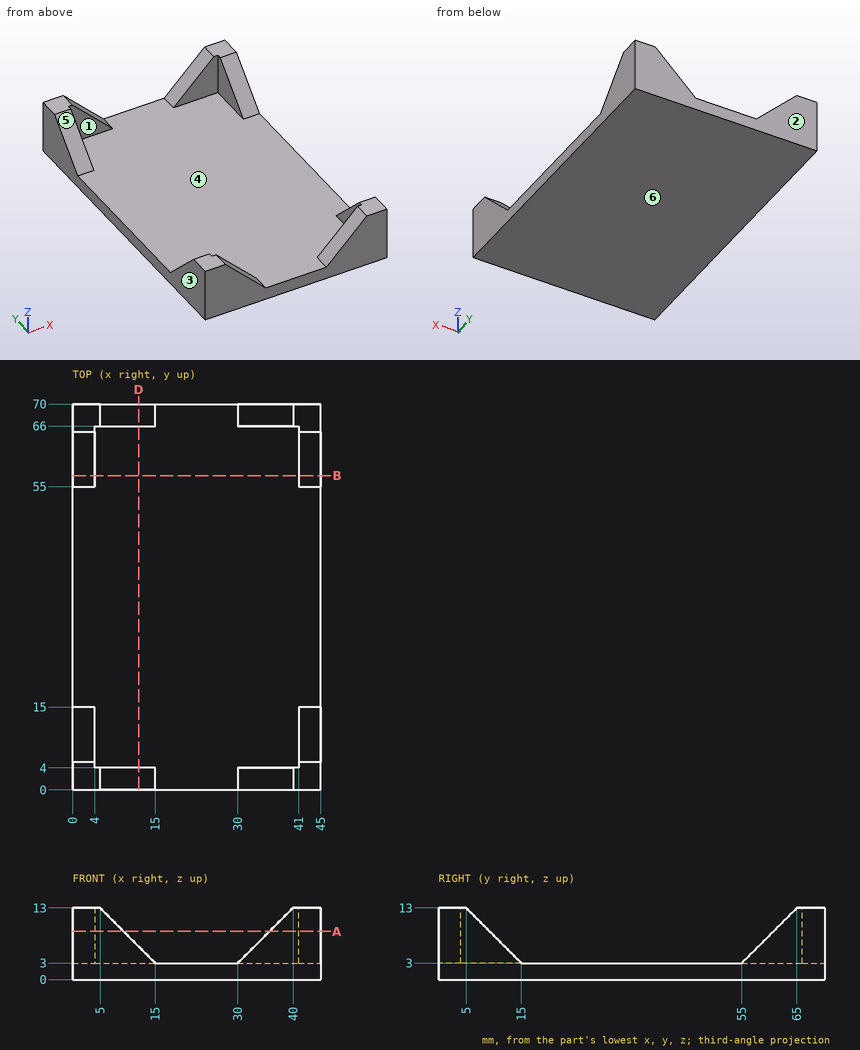
Source: three-view drawing plus pictorial views. Frame: mm from the lowest corner of the part. A direction names the side the tool comes from. Give positions to 0.01 mm unless a question says otherwise; leave off trailing zeros. Write each loop counter-clockwise with the first axis right and the second up, starting at its lowest first coordinate (ties: lowest second). Pieces come first, ordered by that corner, then holes. Notation, with made-up numbers: (50.5, -8.75) - (75.5, -8.75) arc R21 cw to (75.5, 30.25) - close; hole circle Ø3 at (-26, 23). An arc over 180 degrees is marked (long way). Write item = value, one per line. Start each with the question number.
Q1. Pin query (flat end, axial travel): pin 1 Ø2 at (x, z) = (11, 9.5) entering from +Y; pin 2 Ø5 at (x, z) = (5.5, 8) entering from -Y. Return the tip coordinate at first contact, or that it passes through.
Q2. Material intervals for probe 1 along Y at (x, z) = (10, 7); probe 2 along Z at (x, y) = (40, 37); probe 3 along X at (y, z) = (65, 6), sorted ascending.
Q3. Cut plane A-A, the plane z = 8.75. Return loops of the section in (x, y), then the cut area to 3 significant figures.
Q4. Cut plane D-D, the plane x = 12. Return loops of the section in (y, z).
Q5. Draft query along X for the marked faces 1, 2 and 3. Return one class per face: +X half, -X half, draft (parallel to the pull), parting line (faces both ways), or undercut.
Q6. Reachability of the marked faces 4, 5 and 6 from +Z, -Z, +X, -X, +Y, -Y: full face, straight path, thin tool, end or side. Return the list, or none.
Q7. Cut plane B-B, the plane y = 57. Return loops of the section in (x, z), then the cut area to 3 significant figures.
Computed values:
q1.pin_1 = through
q1.pin_2 = 0
q2.probe_1 = 0 to 4, 66 to 70
q2.probe_2 = 0 to 3
q2.probe_3 = 0 to 4, 41 to 45
q3.outline = (0, 0) - (9.25, 0) - (9.25, 4) - (4, 4) - (4, 9.25) - (0, 9.25) - close; (0, 60.75) - (4, 60.75) - (4, 66) - (9.25, 66) - (9.25, 70) - (0, 70) - close; (35.75, 0) - (45, 0) - (45, 9.25) - (41, 9.25) - (41, 4) - (35.75, 4) - close; (35.75, 66) - (41, 66) - (41, 60.75) - (45, 60.75) - (45, 70) - (35.75, 70) - close
q3.area = 232 mm²
q4.outline = (0, 0) - (70, 0) - (70, 6) - (66, 6) - (66, 3) - (4, 3) - (4, 6) - (0, 6) - close
q5.face_1 = undercut
q5.face_2 = draft
q5.face_3 = -X half
q6.face_4 = +Z
q6.face_5 = +Z, +X, -X
q6.face_6 = -Z, +X, -X, +Y, -Y
q7.outline = (0, 0) - (45, 0) - (45, 5) - (41, 5) - (41, 3) - (4, 3) - (4, 5) - (0, 5) - close
q7.area = 151 mm²
